Autodesk Inventor part; units mm, degrees
ref_plane "YZ Plane" through (0, 0, 0) normal (1, 0, 0) x (0, 1, 0)
ref_plane "XZ Plane" through (0, 0, 0) normal (0, 1, 0) x (-1, 0, 0)
ref_plane "XY Plane" through (0, 0, 0) normal (0, 0, 1) x (1, 0, 0)
sketch "Sketch1" plane through (0, 0, 0) normal (0, 1, 0) x (-1, 0, 0)
  line L0 (-11.43, 18.1) -> (11.43, 18.1)
  line L1 (11.43, 18.1) -> (11.43, -18.1)
  line L2 (11.43, -18.1) -> (-11.43, -18.1)
  line L3 (-11.43, -18.1) -> (-11.43, 18.1)
  line L4 (-11.43, 18.1) -> (11.43, -18.1) construction
  line L5 (11.43, 18.1) -> (-11.43, -18.1) construction
  line L6 (-8.825, 15.5) -> (8.825, 15.5) construction
  line L7 (8.825, 15.5) -> (8.825, -15.5) construction
  line L8 (8.825, -15.5) -> (-8.825, -15.5) construction
  line L9 (-8.825, -15.5) -> (-8.825, 15.5) construction
  line L10 (-8.825, 15.5) -> (8.825, -15.5) construction
  line L11 (8.825, 15.5) -> (-8.825, -15.5) construction
  circle A0 centre (8.825, 15.5) radius 1
  circle A1 centre (-8.825, 15.5) radius 1
  circle A2 centre (6.5, -15.5) radius 1
  line L12 (0, 0) -> (0, -18.1)
  circle A3 centre (-6.5, -15.5) radius 1
  dimension "d0" = 22.86
  dimension "d1" = 36.2
  dimension "d2" = 17.65
  dimension "d3" = 31
  dimension "d4" = 6.5
  dimension "d5" = 2
  dimension "d6" = 2
  dimension "d7" = 2
extrude "Extrusion1" add sketch "Sketch1" along normal blind 2
sketch "Sketch2" plane through (0, 2, 0) normal (0, 1, 0) x (1, 0, 0)
  line L0 (-11.43, 18.1) -> (11.3685, 18.1) construction
  line L1 (11.3685, 18.1) -> (11.3685, -18.1704) construction
  line L2 (11.3685, -18.1704) -> (-11.43, -18.1704) construction
  line L3 (-11.43, -18.1704) -> (-11.43, 18.1) construction
  point P0 (0, 0)
decal "Decal1"
properties part number "powerboost"
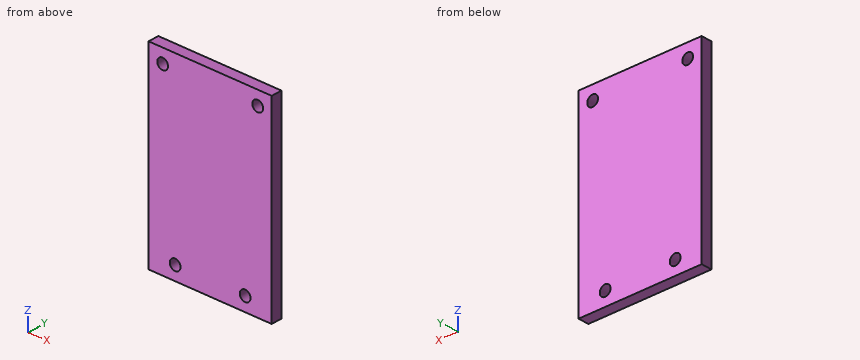
Read the model definition and answer for the solid it produces. Units are mm, in the model's axes. Coordinates: 2 decimals unless noted, no trailing zeros. Order: outer loops, then holes, each group sorted by start corner. A loop starts at its lowest first (then second) coordinate and runs counter-clockwise, first axis right, second up. Notation, with made-up numbers: (61.25, 86.5) - (98.25, 86.5) arc R28 cw to (98.25, 124.5) - close; hole circle Ø1 at (-29.75, 11.5). An arc over 180 degrees is marked (long way). Answer as a JSON object with one key per item and string values. Group by question number.
Item 1: Section B-B (z = 15.5) is taken. Give the vertices of the cut face in (x, y) (3 decimals), plus the area to 3 significant figures.
Item 2: Section D-D (x = 9.25) is taken. Give the vertices of the cut face in (y, z).
Item 3: Section A-A (x = 6.5) is taken. Give the vertices of the cut face in (y, z).
Item 4: Consider probe 1 along Z at (x, y) = (6.5, 1.5); probe 2 along Z at (x, y) = (5.75, 0.65). Determine where each line is inside the solid, lowest interval first. Write a range as from..to.
Item 5: Section C-C (y = 1.35) is taken. Give the vertices of the cut face in (x, z) (3 decimals).
Results are:
{
 "1": {"outline": "(-11.43, 0) - (-9.825, 0) - (-9.825, 2) - (-11.43, 2) - close; (-7.825, 0) - (7.825, 0) - (7.825, 2) - (-7.825, 2) - close; (9.825, 0) - (11.43, 0) - (11.43, 2) - (9.825, 2) - close", "area": "37.7 mm^2"},
 "2": {"outline": "(0, -18.1) - (2, -18.1) - (2, 14.59) - (0, 14.59) - close; (0, 16.41) - (2, 16.41) - (2, 18.1) - (0, 18.1) - close"},
 "3": {"outline": "(0, -18.1) - (2, -18.1) - (2, -16.5) - (0, -16.5) - close; (0, -14.5) - (2, -14.5) - (2, 18.1) - (0, 18.1) - close"},
 "4": {"probe 1": "z = -18.1..-16.5, -14.5..18.1", "probe 2": "z = -18.1..-16.16, -14.84..18.1"},
 "5": {"outline": "(-11.43, -18.1) - (11.43, -18.1) - (11.43, 18.1) - (-11.43, 18.1) - close; hole circle Ø2 at (-8.825, 15.5); hole circle Ø2 at (-6.5, -15.5); hole circle Ø2 at (6.5, -15.5); hole circle Ø2 at (8.825, 15.5)"}
}
